Geometry check sheet. Reference: the model listing, model coordinates, mm. A direction names the side the tool comes from. Round coordinates to 2 decimals unless told otherwise and drop trailing zeros. Write each loop counter-clockwise with the first axis right and the second up, starting at its lowest first coordinate (ties: lowest second). Pieces come first, ordered by that corner, then holes. Notation, with made-up numbers: M 34.5,56 L 38.5,56 A4 ccw 38.5,60 Z; hole C 64.25,62.5 d1. An arc over 180 degrees is marked long. Answer in a Markdown table with one row per item. Add a question column.
from build123d import *

# Parameters (mm, degrees)
EXTRUDE_1_DEPTH     = 5
EXTRUDE_START       = -13.5
EXTRUDE_2_DEPTH     = 8.5
SKETCH_3_R          = 2.75
EXTRUDE_3_DEPTH     = 3
SKETCH_4_R          = 1.45
CUT_EXTRUDE_1_DEPTH = 7


with BuildPart() as part:
    # Эскиз1 → Бобышка-Вытянуть1 (new body)
    with BuildSketch(Plane.XY):
        with BuildLine():
            Line((-20, 3.75), (-20, -3.75))
            Line((-20, -3.75), (-3.225194693, -9.465628304))
            ThreePointArc((-3.225194693, -9.465628304), (10, 0), (-3.225194693, 9.465628304))
            Line((-3.225194693, 9.465628304), (-20, 3.75))
        make_face()
        with BuildLine():
            Line((1.8, 5.708755266), (1.8, 6.512045083))
            ThreePointArc((1.8, 6.512045083), (3.1e-08, 8.312045083), (-1.8, 6.512045145))
            Line((-1.8, 6.512045145), (-1.8, 5.679024933))
            ThreePointArc((-1.8, 5.679024933), (-2.30564415, 4.349776802), (-3.566900594, 3.692655212))
            Line((-3.566900594, 3.692655212), (-15.568064288, 2.284325182))
            ThreePointArc((-15.568064288, 2.284325182), (-17.6, 9e-09), (-15.568064305, -2.28432518))
            Line((-15.568064305, -2.28432518), (-3.566900604, -3.692655149))
            ThreePointArc((-3.566900604, -3.692655149), (-2.305644154, -4.349776736), (-1.8, -5.679024871))
            Line((-1.8, -5.679024871), (-1.8, -6.512045083))
            ThreePointArc((-1.8, -6.512045083), (0, -8.312045083), (1.8, -6.512045083))
            Line((1.8, -6.512045083), (1.8, -5.708755266))
            ThreePointArc((1.8, -5.708755266), (2.036985071, -4.764415094), (2.691778361, -4.043869445))
            ThreePointArc((2.691778361, -4.043869445), (4.857833965, 0), (2.691778361, 4.043869445))
            ThreePointArc((2.691778361, 4.043869445), (2.036985071, 4.764415094), (1.8, 5.708755266))
        make_face(mode=Mode.SUBTRACT)
    extrude(amount=EXTRUDE_1_DEPTH)

    # Эскиз2 → Бобышка-Вытянуть2 (add)
    with BuildSketch(Plane.XY.offset(5).offset(EXTRUDE_START)):
        with BuildLine():
            Line((-3.225194693, 9.465628304), (-20, 3.75))
            Line((-20, 3.75), (-20, -3.75))
            Line((-20, -3.75), (-3.225194693, -9.465628304))
            ThreePointArc((-3.225194693, -9.465628304), (10, 0), (-3.225194693, 9.465628304))
        make_face()
    extrude(amount=EXTRUDE_2_DEPTH)

    # Эскиз3 → Бобышка-Вытянуть3 (add)
    with BuildSketch(Plane(origin=(0, 0, -8.5), x_dir=(-1, 0, 0), z_dir=(0, 0, -1))):
        with Locations(Location((0, 0, 0), (0, 0, 180))):
            Circle(SKETCH_3_R)
    extrude(amount=EXTRUDE_3_DEPTH)

    # Эскиз4 → Вырез-Вытянуть1 (cut)
    with BuildSketch(Plane.ZY.offset(20)):
        with Locations((-5.5, 0)):
            Circle(SKETCH_4_R)
        with Locations((2, 0)):
            Circle(SKETCH_4_R)
    extrude(amount=-CUT_EXTRUDE_1_DEPTH, mode=Mode.SUBTRACT)


solid = part.part
Item 1: Scan lines: probe 1 along Y at (x, z) = (-10, 2.75); probe 2 along Y at (x, z) = (-16, -5.5); probe 3 along Z at (x, y) = (-11, -2). Record each from-to range of solid material in increasing order. Write a range as from..to.
Item 2: Section check B-B, the plane x = 0. Record the boundary of the cut face in (y, z).
Item 3: Section check D-D, the plane x = -16.5. Record the boundary of the cut face in (y, z), and give its area (3 significant figures).
Item 4: Gauge pin test, flat ends, axial feed: pin 1 Ø6 at (x, z) = (-10, -6.5) entering from +Y; pin 2 Ø8 at (y, z) = (4.5, -8.5) entering from +X; pin 3 Ø5 at (y, z) = (6.5, -5) entering from +X. Record the tip position at first contact, or that the pin passes through.
Item 5: Section check A-A, the plane y = 0. Record the boundary of the cut face in (x, z).
Item 6: Section check C-C, the plane z = -5.5. Record the boundary of the cut face in (x, y).
Item 7: Mould release check, pull along X, two halves, no side actions. Record for faces 1 (the flat face through (0, 0, -11.5)), 2 (the cylindrical face through (-0.596, 2.685, -9.979)), 3 (the cylindrical face through (-0.04, -8.31, 2.46)), 4 (the flat face through (-11.495, 6.648, -1.844)): +X half, -X half, draft (parallel to the pull), parting line (faces both ways), or undercut.
Item 8: Access from +Z, -Z, +X, -X, +Y, -Y to the whole of each face (thin tool, end or side, straight path). Record for faces 5 (the flat face through (-1.8, -6, 2)), 6 (the flat face through (-5, 0, -8.5)), 7 (the flat face through (-13, 0, -6)).
Result sheet:
| question | item | result |
|---|---|---|
| 1 | probe 1 | y = -7.16..-2.94, 2.94..7.16 |
| 1 | probe 2 | y = -5.11..-1.45, 1.45..5.11 |
| 1 | probe 3 | z = -8.5..0 |
| 2 | outline | M -10,-8.5 L -2.75,-8.5 L -2.75,-11.5 L 2.75,-11.5 L 2.75,-8.5 L 10,-8.5 L 10,5 L 8.31,5 L 8.31,0 L -8.31,0 L -8.31,5 L -10,5 Z |
| 3 | outline | M -4.94,-8.5 L 4.94,-8.5 L 4.94,5 L 1.96,5 L 1.96,0 L -1.96,0 L -1.96,5 L -4.94,5 Z; hole C 0,-5.5 d2.9 |
| 3 | area | 107 mm^2 |
| 4 | pin 1 | stops at y = 8.18 |
| 4 | pin 2 | stops at x = 9.99 |
| 4 | pin 3 | stops at x = 9.17 |
| 5 | outline | M -20,-8.5 L -2.75,-8.5 L -2.75,-11.5 L 2.75,-11.5 L 2.75,-8.5 L 10,-8.5 L 10,5 L 4.86,5 L 4.86,0 L -17.6,0 L -17.6,0.55 L -20,0.55 L -20,-4.05 L -13,-4.05 L -13,-6.95 L -20,-6.95 Z; M -20,3.45 L -17.6,3.45 L -17.6,5 L -20,5 Z |
| 6 | outline | M -20,-3.75 L -3.23,-9.47 A10 ccw long -3.23,9.47 L -20,3.75 L -20,1.45 L -13,1.45 L -13,-1.45 L -20,-1.45 Z |
| 7 | face 1 | draft |
| 7 | face 2 | parting line |
| 7 | face 3 | undercut |
| 7 | face 4 | -X half |
| 8 | face 5 | +Z |
| 8 | face 6 | -Z |
| 8 | face 7 | -X |
